Can you work these out from the model? Positions are in its coordinate system, mm. A direction names the side the tool comes from. Round coordinates to 2 decimals unless told otherwise and drop trailing zeros. Order: outer loops, then holes, each group sorted by start corner. A loop starts at its lowest first (then second) coordinate and runs counter-clockwise, first axis right, second up.
Q1. If we section it at B-B (z = 5): Please give me the cut outline in (x, y), plus the area to 3 significant figures.
Q2. For faces 5 (the face through (124.044, 10.693, 6.038)), 6 (the face through (-58.956, 10.693, 6.038)), 7 (the face through (33, 2.689, 5)), 8 (the face through (122.565, 9, 5)), which set-ups out of +Z, -Z, +X, -X, +Y, -Y let a thin tool reach every point of the face, with its end or its side?
Q3. If we section it at C-C (x = 26): Please give me the cut outline in (y, z).
Q4. If I drill on line 1 (X direction, y = 13.5, z = 1.5); line 2 (Y direction, x = -58.4, z = 5); line 3 (Y direction, x = 11, z = 5.5), over which ranges is the centre line in solid material (lowest first)?
Q5. We'd pull the mould along X, two halves only. Please class faces 1 (the face through (125.565, 15.1, 4.9)), 2 (the face through (-57.435, 9, 5)), 3 (the face through (31, 22.689, 5)), 4 (the face through (37.565, 11, 5)): pulls with the +X half, pulls with the -X half, needs draft (parallel to the pull), parting line crosses it, or undercut.
Q6. Will this pin go through, and if not, where does the flat tip stop? P1, Ø1, axis at x = -5.5, z = 5, coming from the -Y side.
Q7. If we section it at A-A (y = 16.5): Please give me the cut outline in (x, z), plus the area to 3 significant figures.
from build123d import *

# Parameters (mm, degrees)
DODANIE_WYCI_GNI_CIE1_DEPTH = 10
SZKIC4_R                    = 2.25
WYTNIJ_WYCI_GNI_CIE1_DEPTH  = 10
WYTNIJ_WYCI_GNI_CIE2_START  = -183
SZKIC4_2_R                  = 2.25
WYTNIJ_WYCI_GNI_CIE2_DEPTH  = 10


with BuildPart() as part:
    # Szkic2 → Dodanie-wyciągnięcie1 (new body)
    with BuildSketch(Plane.XY):
        Polygon((-60.434598082, 22.68907563), (125.565401918, 22.68907563), (125.565401918, 2.68907563), (122.565401918, 2.68907563), (122.565401918, 19.68907563), (37.565401918, 19.68907563), (37.565401918, 2.68907563), (27.565401918, 2.68907563), (27.565401918, 19.68907563), (-57.434598082, 19.68907563), (-57.434598082, 2.68907563), (-60.434598082, 2.68907563), align=None)
    extrude(amount=DODANIE_WYCI_GNI_CIE1_DEPTH)

    # Szkic4 → Wytnij-wyciągnięcie1 (cut)
    with BuildSketch(Plane.ZY.offset(60.434598082)):
        with Locations((5, 12.68907563)):
            Circle(SZKIC4_R)
    extrude(amount=-WYTNIJ_WYCI_GNI_CIE1_DEPTH, mode=Mode.SUBTRACT)

    # Szkic4<2> → Wytnij-wyciągnięcie2 (cut)
    with BuildSketch(Plane.ZY.offset(60.434598082).offset(WYTNIJ_WYCI_GNI_CIE2_START)):
        with Locations((5, 12.68907563)):
            Circle(SZKIC4_2_R)
    extrude(amount=-WYTNIJ_WYCI_GNI_CIE2_DEPTH, mode=Mode.SUBTRACT)


solid = part.part
Solution:
1. outline: (-60.43, 2.69) - (-57.43, 2.69) - (-57.43, 10.44) - (-60.43, 10.44) - close; (-60.43, 14.94) - (-57.43, 14.94) - (-57.43, 19.69) - (27.57, 19.69) - (27.57, 2.69) - (37.57, 2.69) - (37.57, 19.69) - (122.57, 19.69) - (122.57, 14.94) - (125.57, 14.94) - (125.57, 22.69) - (-60.43, 22.69) - close; (122.57, 2.69) - (125.57, 2.69) - (125.57, 10.44) - (122.57, 10.44) - close
1. area: 803 mm2
2. face 5: +X
2. face 6: -X
2. face 7: +Z, -Z, +X, -X, -Y
2. face 8: +Z, -Z, -Y
3. outline: (19.69, 0) - (22.69, 0) - (22.69, 10) - (19.69, 10) - close
4. line 1: x = -60.43 to -57.43, 27.57 to 37.57, 122.57 to 125.57
4. line 2: y = 2.69 to 10.44, 14.94 to 22.69
4. line 3: y = 19.69 to 22.69
5. face 1: pulls with the +X half
5. face 2: undercut
5. face 3: needs draft
5. face 4: undercut
6. P1: stops at y = 19.69
7. outline: (-60.43, 0) - (-57.43, 0) - (-57.43, 10) - (-60.43, 10) - close; (27.57, 0) - (37.57, 0) - (37.57, 10) - (27.57, 10) - close; (122.57, 0) - (125.57, 0) - (125.57, 10) - (122.57, 10) - close
7. area: 160 mm2
